Read the model definition and answer for the solid it produces. Units are mm, in the model's axes. Coordinates: 2 decimals unless noted, no trailing zeros. Loops run counter-clockwise (first coordinate to the right, second up) from the corner with the lowest first, then second, coordinate; pieces in that order, holes last. Notation, with made-up numbers: (28.25, 51.25) -> (70.25, 51.25) arc R23 cw to (70.25, 89.25) -> close; hole circle Ø4 at (-31.5, -3.5). An arc over 180 degrees is marked (long way). Answer as CSV lines item,"result".
```python
from build123d import *

# Parameters (mm, degrees)
F1_DEPTH = 5


with BuildPart() as f1:
    # F0 (on Top) → F1 (new body)
    with BuildSketch(Plane.XY):
        with BuildLine():
            ThreePointArc((-49.3595098916, 110.2112788137), (-84.71847747, 94.422814407), (-112.0164757766, 66.9573545531))
            ThreePointArc((-112.0164757766, 66.9573545531), (-111.4379878132, 62.359119868), (-107.33126292, 60.2112788137))
            ThreePointArc((-107.33126292, 60.2112788137), (-99.8206092018, 62.444259798), (-92.3099554835, 60.2112788137))
            Line((-92.3099554835, 60.2112788137), (0, 0))
            Line((0, 0), (-110.2112788137, 0))
            ThreePointArc((-110.2112788137, 0), (-109.0627736394, -15.869385112), (-105.6411951245, -31.4080223893))
            ThreePointArc((-105.6411951245, -31.4080223893), (-100.0178554155, -46.292057373), (-92.3099554835, -60.2112788137))
            ThreePointArc((-92.3099554835, -60.2112788137), (-99.8206092018, -62.444259798), (-107.33126292, -60.2112788137))
            ThreePointArc((-107.33126292, -60.2112788137), (-111.4379878132, -62.359119868), (-112.0164757766, -66.9573545531))
            ThreePointArc((-112.0164757766, -66.9573545531), (-62.7481057699, -106.0388311627), (0, -110.2112788137))
            ThreePointArc((0, -110.2112788137), (62.7481057699, -106.0388311627), (112.0164757766, -66.9573545531))
            ThreePointArc((112.0164757766, -66.9573545531), (111.4379878132, -62.359119868), (107.33126292, -60.2112788137))
            ThreePointArc((107.33126292, -60.2112788137), (99.8206092018, -62.444259798), (92.3099554835, -60.2112788137))
            ThreePointArc((92.3099554835, -60.2112788137), (100.0178554155, -46.292057373), (105.6411951245, -31.4080223893))
            ThreePointArc((105.6411951245, -31.4080223893), (109.0627736394, -15.869385112), (110.2112788137, 0))
            ThreePointArc((110.2112788137, 0), (109.0627736394, 15.869385112), (105.6411951245, 31.4080223893))
            ThreePointArc((105.6411951245, 31.4080223893), (100.0178554155, 46.292057373), (92.3099554835, 60.2112788137))
            ThreePointArc((92.3099554835, 60.2112788137), (99.8206092018, 62.444259798), (107.33126292, 60.2112788137))
            ThreePointArc((107.33126292, 60.2112788137), (110.1834218657, 61.1045539205), (112.0164757766, 63.4652030743))
            Line((112.0164757766, 63.4652030743), (112.0164757766, 66.9573545531))
            ThreePointArc((112.0164757766, 66.9573545531), (84.71847747, 94.422814407), (49.3595098916, 110.2112788137))
            Line((49.3595098916, 110.2112788137), (0, 110.2112788137))
            Line((0, 110.2112788137), (-49.3595098916, 110.2112788137))
        make_face()
        with BuildLine():
            ThreePointArc((-17.676910541, 82.5358693145), (-12.9316790716, 94.5842825427), (-1.2471505461, 100.165794538))
            Line((-1.2471505461, 100.165794538), (-1.2471505461, 82.5358693145))
            Line((-1.2471505461, 82.5358693145), (-1.2471505461, 65.0322264722))
            Line((-1.2471505461, 65.0322264722), (-1.2471505461, 64.8986584064))
            ThreePointArc((-1.2471505461, 64.8986584064), (-3.2688897914, 65.1595640594), (-5.2471505461, 65.6514845023))
            Line((-5.2471505461, 65.6514845023), (-5.2471505461, 91.2374200697))
            Line((-5.2471505461, 91.2374200697), (-5.2471505461, 91.3882628083))
            ThreePointArc((-5.2471505461, 91.3882628083), (-5.4893133361, 91.7531337591), (-5.9247359984, 91.7998320749))
            ThreePointArc((-5.9247359984, 91.7998320749), (-6.030968486, 91.7310453203), (-6.1364025444, 91.6610409037))
            ThreePointArc((-6.1364025444, 91.6610409037), (-9.7068547443, 87.705450119), (-10.9992407835, 82.5358693145))
            Line((-10.9992407835, 82.5358693145), (-17.676910541, 82.5358693145))
        make_face(mode=Mode.SUBTRACT)
        with BuildLine():
            Line((17.6757126889, 82.222390346), (5.25, 82.222390346))
            Line((5.25, 82.222390346), (5.25, 65.6518987247))
            ThreePointArc((5.25, 65.6518987247), (3.2717488011, 65.1598166454), (1.25, 64.8987527373))
            Line((1.25, 64.8987527373), (1.25, 65.0322264722))
            Line((1.25, 65.0322264722), (1.25, 82.5322264722))
            Line((1.25, 82.5322264722), (1.25, 100.165700207))
            ThreePointArc((1.25, 100.165700207), (13.0400026737, 94.4686461336), (17.6757126889, 82.222390346))
        make_face(mode=Mode.SUBTRACT)
        with BuildLine():
            ThreePointArc((0, 110.2112788137), (-24.6797549458, 113.1333968343), (-49.3595098916, 110.2112788137))
            Line((-49.3595098916, 110.2112788137), (0, 110.2112788137))
        make_face()
        with BuildLine():
            Line((0, 0), (-92.3099554835, 60.2112788137))
            ThreePointArc((-92.3099554835, 60.2112788137), (-96.4154183349, 53.3909457218), (-100.0178554155, 46.292057373))
            Line((-100.0178554155, 46.292057373), (0, 0))
        make_face()
        with BuildLine():
            ThreePointArc((49.3595098916, 110.2112788137), (24.6797549458, 113.1333968343), (0, 110.2112788137))
            Line((0, 110.2112788137), (49.3595098916, 110.2112788137))
        make_face()
        with BuildLine():
            Line((0, 0), (-100.0178554155, 46.292057373))
            ThreePointArc((-100.0178554155, 46.292057373), (-103.09847182, 38.9516506215), (-105.6411951245, 31.4080223893))
            Line((-105.6411951245, 31.4080223893), (0, 0))
        make_face()
        with BuildLine():
            Line((-109.0627736443, 15.869385078), (0, 0))
            Line((0, 0), (-105.6411951245, 31.4080223893))
            ThreePointArc((-105.6411951245, 31.4080223893), (-107.6327592495, 23.7005298274), (-109.0627736443, 15.869385078))
        make_face()
        with BuildLine():
            Line((-110.2112788137, 0), (0, 0))
            Line((0, 0), (-109.0627736443, 15.869385078))
            ThreePointArc((-109.0627736443, 15.869385078), (-109.923777528, 7.955445413), (-110.2112788137, 0))
        make_face()
        with BuildLine():
            ThreePointArc((-109.0627736443, 15.869385078), (-107.6327592495, 23.7005298274), (-105.6411951245, 31.4080223893))
            ThreePointArc((-105.6411951245, 31.4080223893), (-112.2040526288, 35.6887962365), (-115.362225006, 42.8597146287))
            ThreePointArc((-115.362225006, 42.8597146287), (-120.874929791, 44.3257734811), (-124.1738093645, 39.6721043733))
            ThreePointArc((-124.1738093645, 39.6721043733), (-120.0946527482, 18.8146599148), (-110.2112788137, 0))
            ThreePointArc((-110.2112788137, 0), (-109.923777528, 7.955445413), (-109.0627736443, 15.869385078))
        make_face()
        with BuildLine():
            ThreePointArc((-105.6411951245, -31.4080223893), (-109.0627736394, -15.869385112), (-110.2112788137, 0))
            ThreePointArc((-110.2112788137, 0), (-120.0946527482, -18.8146599148), (-124.1738093645, -39.6721043733))
            ThreePointArc((-124.1738093645, -39.6721043733), (-120.874929791, -44.3257734811), (-115.362225006, -42.8597146287))
            ThreePointArc((-115.362225006, -42.8597146287), (-112.2040526288, -35.6887962365), (-105.6411951245, -31.4080223893))
        make_face()
        with BuildLine():
            ThreePointArc((112.0164757766, 63.4652030743), (112.33126292, 65.2112788137), (112.0164757766, 66.9573545531))
            Line((112.0164757766, 66.9573545531), (112.0164757766, 63.4652030743))
        make_face()
        with BuildLine():
            ThreePointArc((115.362225006, 42.8597146287), (112.2040526288, 35.6887962365), (105.6411951245, 31.4080223893))
            ThreePointArc((105.6411951245, 31.4080223893), (109.0627736394, 15.869385112), (110.2112788137, 0))
            ThreePointArc((110.2112788137, 0), (120.0946527482, 18.8146599148), (124.1738093645, 39.6721043733))
            ThreePointArc((124.1738093645, 39.6721043733), (120.874929791, 44.3257734811), (115.362225006, 42.8597146287))
        make_face()
        with BuildLine():
            ThreePointArc((124.1738093645, -39.6721043733), (120.0946527482, -18.8146599148), (110.2112788137, 0))
            ThreePointArc((110.2112788137, 0), (109.0627736394, -15.869385112), (105.6411951245, -31.4080223893))
            ThreePointArc((105.6411951245, -31.4080223893), (112.2040526288, -35.6887962365), (115.362225006, -42.8597146287))
            ThreePointArc((115.362225006, -42.8597146287), (120.874929791, -44.3257734811), (124.1738093645, -39.6721043733))
        make_face()
    extrude(amount=F1_DEPTH)


solid = f1.part
```
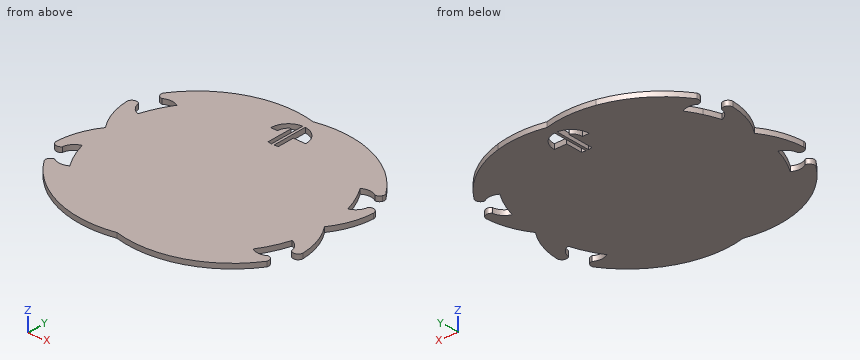
Q1. Find the intervals of material crossed by probe 1 along X at (y, z) = (73, 1.2); probe 2 along X at (y, z) = (98.5, 2.05); probe 3 along Y at (x, z) = (-99, 0.95), in increasing order. Write a range as [from, to].
Results:
probe 1,"x = [-107.58, -5.25], [-1.25, 1.25], [5.25, 107.58]"
probe 2,"x = [-78.33, -7.58], [-1.25, 1.25], [7.59, 78.33]"
probe 3,"y = [-82.59, -62.42], [-48.43, 48.43], [62.42, 82.59]"
Q2. A cutting plane is placed at A-A, the plane z = 0.75. Give the number of separate pieces and of enclosed holes in the cut face, and give its area (3 significant figures).
Results:
separate pieces,"1"
enclosed holes,"2"
area,"45,100 mm²"
Q3. Given pin 1 Ø1.5 at (y, z) = (90.5, 2.5) entering from -X; pin 2 Ø1 at (x, z) = (-58.5, 2) entering from -Y; pin 3 Ø1.5 at (y, z) = (81, 3.5) entering from +X, each flat-ended and moving along its own axis, determine where each tip first touches the part or whether it passes through.
Results:
pin 1,"stops at x = -90.98"
pin 2,"stops at y = -107.74"
pin 3,"stops at x = 101.29"
Q4. A cutting plane is placed at B-B, the plane y = -10. Write down the section's boundary in (x, z), and give its area (3 significant figures).
Results:
outline,"(-116.33, 0) -> (116.33, 0) -> (116.33, 5) -> (-116.33, 5) -> close"
area,"1,160 mm²"
Q5. A cutting plane is placed at C-C, the plane x = 63.5. Write down the section's boundary in (y, z), and give its area (3 significant figures).
Results:
outline,"(-105.75, 0) -> (105.75, 0) -> (105.75, 5) -> (-105.75, 5) -> close"
area,"1,060 mm²"
